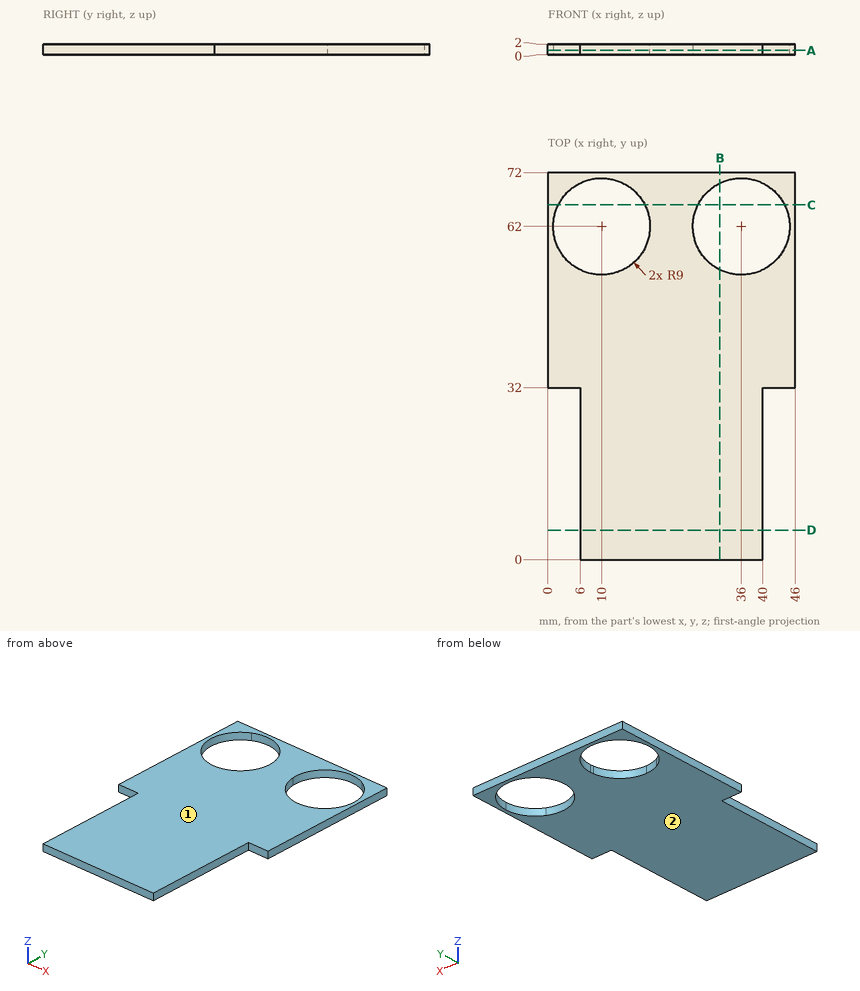
Study the drawing (mm; zero at the part's minimum x, y, z) and answer. Round coordinates to 2 decimals unless told otherwise and drop trailing zeros. Order: outer loops, then holes, each group sorted by start corner. A loop starts at its lowest first (then second) coordinate and runs counter-clockwise, first axis right, second up. Notation, with made-up numbers: (40.5, 9) -> (88.5, 9) arc R20 cw to (88.5, 30) -> close; hole circle Ø11 at (51, -0.5). An arc over 180 degrees is marked (long way). Answer as CSV lines item,"result". Start each with the question number.
(1) The part is cut by section A-A (z = 0.8). Determine the outline of the cut face in (x, y).
(2) For a pull along Z with two mould halves and no side action, classify the marked faces 1 and 2 as +Z half, -Z half, draft (parallel to the pull), parting line (faces both ways), or undercut.
(3) The part is cut by section B-B (x = 32). Determine the outline of the cut face in (y, z), then the cut area to 3 significant figures.
(4) Flat-ended cylindrical pins translate along their axes: pin 1 Ø1 at (x, z) = (3, 1.5) entering from -Y; pin 2 Ø4 at (x, y) = (37.5, 42.5) entering from -Z; pin 3 Ø1 at (y, z) = (23, 0.5) entering from -X; pin 4 Ø0.6 at (y, z) = (12, 1.5) entering from +X. Find the tip coordinate at first contact, or state that the pin passes through.
(5) The part is cut by section C-C (y = 66). Determine the outline of the cut face in (x, z).
(6) The part is cut by section D-D (y = 5.5). Determine the outline of the cut face in (x, z).
(7) Find the intervals of material crossed by probe 1 along X at (y, z) = (63.5, 1.3); probe 2 along Y at (x, z) = (10.5, 0.65); probe 3 along Y at (x, z) = (38, 0.9), in increasing order. Write a range as from..to.
Evaluation:
1,outline,"(0, 32) -> (6, 32) -> (6, 0) -> (40, 0) -> (40, 32) -> (46, 32) -> (46, 72) -> (0, 72) -> close; hole circle Ø18 at (10, 62); hole circle Ø18 at (36, 62)"
2,face 1,"+Z half"
2,face 2,"-Z half"
3,outline,"(0, 0) -> (53.94, 0) -> (53.94, 2) -> (0, 2) -> close; (70.06, 0) -> (72, 0) -> (72, 2) -> (70.06, 2) -> close"
3,area,"112 mm²"
4,pin 1,"y = 32"
4,pin 2,"z = 0"
4,pin 3,"x = 6"
4,pin 4,"x = 40"
5,outline,"(0, 0) -> (1.94, 0) -> (1.94, 2) -> (0, 2) -> close; (18.06, 0) -> (27.94, 0) -> (27.94, 2) -> (18.06, 2) -> close; (44.06, 0) -> (46, 0) -> (46, 2) -> (44.06, 2) -> close"
6,outline,"(6, 0) -> (40, 0) -> (40, 2) -> (6, 2) -> close"
7,probe 1,"0..1.13, 18.87..27.13, 44.87..46"
7,probe 2,"0..53.01, 70.99..72"
7,probe 3,"0..53.23, 70.77..72"
